```python
from build123d import *

# Parameters (mm, degrees)
SCHIZZO2_R                   = 17.5
ESTRUSIONE_ESTRUSIONE2_DEPTH = 15
ESTRUSIONE_ESTRUSIONE3_DEPTH = 5
FORO_5_0_5_1_D               = 5
FORO_5_0_5_1_CSINK_D         = 5.05
FORO_5_0_5_1_CSINK_ANGLE     = 90


with BuildPart() as part:
    # Schizzo2 → Estrusione-Estrusione2 (new, symmetric)
    with BuildSketch(Plane.XY):
        Circle(SCHIZZO2_R)
        with BuildLine():
            ThreePointArc((2.5, -10.712142643), (0, 11), (-2.5, -10.712142643))
            Line((-2.5, -10.712142643), (-2.5, -13))
            Line((-2.5, -13), (2.5, -13))
            Line((2.5, -13), (2.5, -10.712142643))
        make_face(mode=Mode.SUBTRACT)
    extrude(amount=ESTRUSIONE_ESTRUSIONE2_DEPTH, both=True)

    # Schizzo2<8> → Estrusione-Estrusione3 (add, symmetric)
    with BuildSketch(Plane.XY):
        with BuildLine():
            Line((-45.722431864, 45.193575035), (-40.722431864, 36.533320997))
            ThreePointArc((-40.722431864, 36.533320997), (-20.917414575, 26.550556749), (-16.843225773, 4.749288954))
            ThreePointArc((-16.843225773, 4.749288954), (-6.591440531, 16.211197109), (8.750000884, 15.155444056))
            ThreePointArc((8.750000884, 15.155444056), (7.731750254, 15.829418494), (6.803236294, 16.62247443))
            Line((6.803236294, 16.62247443), (-19.439551712, 41.966109335))
            ThreePointArc((-19.439551712, 41.966109335), (-32.041033104, 47.97699794), (-45.722431864, 45.193575035))
        make_face()
        with BuildLine():
            ThreePointArc((17.5, 0), (15.268302341, -8.551546271), (9.142406443, -14.922010737))
            ThreePointArc((9.142406443, -14.922010737), (31.890315924, -9.07231341), (54, -17))
            Line((54, -17), (64, -17))
            ThreePointArc((64, -17), (59.47377273, -3.633352456), (47.757521221, 4.233251032))
            Line((47.757521221, 4.233251032), (11.132944899, 14.164220862))
            ThreePointArc((11.132944899, 14.164220862), (9.909360784, 14.582633544), (8.750000884, 15.155444056))
            ThreePointArc((8.750000884, 15.155444056), (15.155444821, 8.749999558), (17.5, 0))
        make_face()
    extrude(amount=ESTRUSIONE_ESTRUSIONE3_DEPTH, both=True)

    # Foro Ø5.0 (5)-1 (through all)
    with Locations(Plane(origin=(-38.892335599, 43.363541782, 5), x_dir=(1, 0, 0), z_dir=(0, 0, 1))):
        with Locations((0, 0), (97.848441208, -55.318294404)):
            CounterSinkHole(FORO_5_0_5_1_D / 2, FORO_5_0_5_1_CSINK_D / 2, counter_sink_angle=FORO_5_0_5_1_CSINK_ANGLE)


solid = part.part
```
Here's how the part is built. I have some questions about the finished solid (model axes, mm). A direction names the side the tool comes from. Give positions to 0.01 mm unless a question says otherwise; leave off trailing zeros. Write each loop counter-clockwise with the first axis right and the second up, starting at its lowest first coordinate (ties: lowest second). Pieces come first, ordered by that corner, then holes.
(1) Imagine slicing it at D-D, the plane x = 14.5. Write out the boundary of the cut face in (y, z), and give its area (3 significant figures).
Output values:
outline: (-12.17, -5) - (-9.8, -5) - (-9.8, -15) - (9.8, -15) - (9.8, -5) - (13.25, -5) - (13.25, 5) - (9.8, 5) - (9.8, 15) - (-9.8, 15) - (-9.8, 5) - (-12.17, 5) - close
area: 646 mm2
(2) On a 3-axis mill with a long thin cutter (end or side, diameter ignored), from which of +Z, -Z, +X, -X, +Y, -Y can I reach the whole of each face in a straight line? I mean faces 5 (the face through (-3.794, -17.084, 0.21)), 6 (the face through (59, -17, 0)), 7 (the face through (-2.5, -12, 0)), 8 (the face through (8, 8, -15)). Say none if no direction works.
Output values:
face 5: none
face 6: +Z, -Z, +X, -Y
face 7: +Z, -Z
face 8: -Z, +X, -X, +Y, -Y
(3) Thinking about a two-plate mould opening in X: for faces 1 (the face through (-21, 31, -5)), 2 (the face through (-43.257, 40.924, 0.07)), 3 (the face through (29.7, 9.13, -0.07)), 4 (the face through (2.5, -12, 0)), which applies, pulls with the +X half, pulls with the -X half, needs draft (parallel to the pull), parting line crosses it, or undercut?
Output values:
face 1: needs draft
face 2: pulls with the -X half
face 3: pulls with the +X half
face 4: undercut
(4) Imagine slicing it at C-C, the plane y = 0. Write out the boundary of the cut face in (x, z).
Output values:
outline: (-17.5, -15) - (-11, -15) - (-11, 15) - (-17.5, 15) - close; (11, -15) - (17.5, -15) - (17.5, -5) - (55.96, -5) - (55.96, 5) - (17.5, 5) - (17.5, 15) - (11, 15) - close
(5) Imagine slicing it at A-A, the plane z = 9.75. Write out the boundary of the cut face in (x, y), and give its area (3 significant figures).
Output values:
outline: circle Ø35 at (0, 0); hole (-2.5, -13) - (2.5, -13) - (2.5, -10.71) arc R11 ccw (long way) to (-2.5, -10.71) - close
area: 572 mm2
(6) Will these pins go through, and if not, where does the flat tip stop? pin 1 (21.5 mm diameter, centred on x = -22, y = 27, fed in from -Z); pin 2 (13 mm diameter, centred on x = -19.5, y = 33, fed in from +Z); pin 3 (12 mm diameter, centred on x = 46, z = -1, fed in from +Y).
Output values:
pin 1: stops at z = -5
pin 2: stops at z = 5
pin 3: stops at y = 6.34
(7) If I drill on L1, parallel to X at y = -12, z = -3.25; L2, parallel to X at y = -5, z = -9.5; L3, parallel to Z at x = -7, y = 25, over which ranges is the centre line in solid material (lowest first)?
Output values:
L1: x = -12.74 to -2.5, 2.5 to 14.91, 45.17 to 56.46, 61.46 to 63.42
L2: x = -16.77 to -9.8, 9.8 to 16.77
L3: z = -5 to 5
(8) Imagine slicing it at B-B, the plane x = 0. Write out the boundary of the cut face in (y, z), and give its area (3 significant figures).
Output values:
outline: (-17.5, -15) - (-13, -15) - (-13, 15) - (-17.5, 15) - close; (11, -15) - (17.5, -15) - (17.5, -5) - (23.19, -5) - (23.19, 5) - (17.5, 5) - (17.5, 15) - (11, 15) - close
area: 387 mm2
